CAD build for the part. Positions are in the model's coordinates, mm. Face numbers are marked on the shaded views. Round coordinates to 2 decimals unless told otherwise and drop trailing zeros. Order: outer loops, then holes, each group sorted by start corner. A loop starts at its lowest first (then second) coordinate and runs counter-clockwise, first axis right, second up. Notation, with made-up numbers: M -20.75,-35.5 L 13.25,-35.5 A27 cw 13.25,-11.5 Z; hole C 3.5,59.25 d2. An arc over 180 degrees is marked long. Put each result on its own line as item: value.
```python
from build123d import *

# Parameters (mm, degrees)
SKETCH3_R           = 14
SKETCH3_R_2         = 11
SKETCH5_R           = 14
SKETCH5_R_2         = 11
BOSS_EXTRUDE1_DEPTH = 33
SKETCH6_R           = 11
CUT_EXTRUDE1_DEPTH  = 53
CUT_EXTRUDE2_START  = -33
SKETCH7_R           = 11
CUT_EXTRUDE2_DEPTH  = 33


with BuildPart() as part:
    # Sweep1: sweep along a path in Sketch1
    with BuildLine(Plane.XY) as sweep1_path:
        Line((32, 0), (-32, 0))
    # Sketch3 → Sweep1 (sweep)
    with BuildSketch(Plane(origin=(32, 0, 0), x_dir=(0, 0, -1), z_dir=(1, 0, 0))):
        Circle(SKETCH3_R)
        Circle(SKETCH3_R_2, mode=Mode.SUBTRACT)
    sweep(path=sweep1_path.line)

    # Sketch5 → Boss-Extrude1 (add)
    with BuildSketch(Plane(origin=(0, 0, 0), x_dir=(1, 0, 0), z_dir=(0, 1, 0))):
        with Locations(Location((0, 0, 0), (0, 0, 270))):
            Circle(SKETCH5_R)
        with Locations(Location((0, 0, 0), (0, 0, 90))):
            Circle(SKETCH5_R_2, mode=Mode.SUBTRACT)
    extrude(amount=BOSS_EXTRUDE1_DEPTH)

    # Sketch6 → Cut-Extrude1 (cut)
    with BuildSketch(Plane.ZY.offset(32)):
        with Locations(Location((0, 0, 0), (0, 0, 180))):
            Circle(SKETCH6_R)
    extrude(amount=-CUT_EXTRUDE1_DEPTH, mode=Mode.SUBTRACT)

    # Sketch7 → Cut-Extrude2 (cut)
    with BuildSketch(Plane(origin=(0, 33, 0), x_dir=(1, 0, 0), z_dir=(0, 1, 0)).offset(CUT_EXTRUDE2_START)):
        with Locations(Location((0, 0, 0), (0, 0, 270))):
            Circle(SKETCH7_R)
    extrude(amount=CUT_EXTRUDE2_DEPTH, mode=Mode.SUBTRACT)


solid = part.part
```
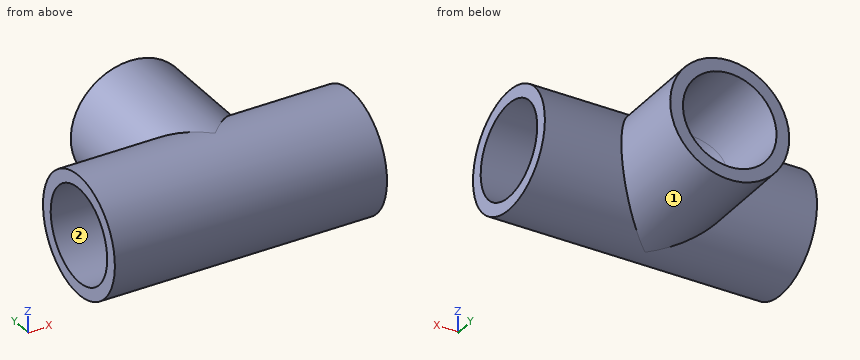
Item 1: Band-saw the part on D-D on y = 28.5. Give the cut face in (x, z), and give its area (3 significant figures).
Answers below:
outline: C 0,0 d28; hole C 0,0 d22
area: 236 mm²
Item 2: Band-saw the part on B-B on y = -2.5. Give the cut face in (x, z).
Answers below:
outline: M -32,-13.77 L 32,-13.77 L 32,-10.71 L -32,-10.71 Z; M -32,10.71 L 32,10.71 L 32,13.77 L -32,13.77 Z
Item 3: Probe line 1 along Z through (x, y) = (0, 5). List the from-to ranges inside material, lowest first. Write a range as [from, to].
Answers below:
line 1: [-14, -11], [11, 14]
Item 4: Band-saw the part on A-A on z = 0. Give the cut face in (x, y).
Answers below:
outline: M -32,-14 L 32,-14 L 32,-11 L -32,-11 Z; M -32,11 L -11,11 L -11,33 L -14,33 L -14,14 L -32,14 Z; M 11,11 L 32,11 L 32,14 L 14,14 L 14,33 L 11,33 Z
Item 5: Mould opens along Z. For the marked faces 1 and 2 say: pulls with the +Z half, pulls with the -Z half, needs draft (parallel to the pull), parting line crosses it, or undercut.
Answers below:
face 1: parting line crosses it
face 2: undercut
Item 6: Pin check, flat tips, straight feed: P1, Ø1, axis at x = -24, z = -1.5, coming from the -Y side; P2, Ø13, axis at x = 0, z = 0, coming from the +Y side; P3, Ø8, axis at x = -15.5, y = -5.5, coming from the -Z side. Stop position of each tip, or through.
Answers below:
P1: y = -13.96
P2: y = -8.87
P3: z = -13.92
Item 7: Band-saw the part on C-C on x = 0. Give the cut face in (y, z).
Answers below:
outline: M 0,-14 L 33,-14 L 33,-11 L 0,-11 A11 cw 0,11 L 33,11 L 33,14 L 0,14 A14 ccw Z
